Can you work these out from the model? Positions are in its coordinate system, mm. Face numbers are marked on the shaded views. A direction names the side the tool comes from. Give positions to 0.01 mm unless a question says otherwise; leave off trailing zeros. Write each loop counter-clockwise with the first axis right and the second up, starting at its lowest first coordinate (ties: lowest second). Pieces come first, ordered by that corner, then holes. Notation, with made-up numbers: (79, -13.75) -> (127, -13.75) arc R11 ccw to (127, 5.25) -> close; hole circle Ø2 at (-16.5, 34.5). An arc over 180 degrees is marked (long way). Answer as CSV lines item,"result". Start each with the question number.
1. If we mould it in two halves opening along Z, with no side actions, what happens to the marked faces 6, 7, 8 and 9? For each: pulls with the +Z half, pulls with the -Z half, needs draft (parallel to the pull), parting line crosses it, or undercut.
2. If we section it at B-B on y = 3.5: Count the separate pieces of the cut face and the enclosed holes in it, plus the area to 3 significant figures.
3. I'm going to push flat-ended pins straight in: P1, Ø0.8, axis at x = 4, y = 13, coming from the -Z side; P2, Ø2, axis at x = 1, z = 10.5, coming from the +Y side. Where does each tip first touch, or does it pass through?
4. On a 3-axis mill with a long thin cutter (end or side, diameter ignored), from which of +Z, -Z, +X, -X, +Y, -Y can I reach the whole of each face in a straight line? I mean the marked faces 1, 2, 3, 4 and 5. Say none if no direction works.
5. I need wall thicknesses on line 1 (X direction, y = 13.25, z = 11.25) (3 decimals); line 2 (Z direction, x = 18, y = 7); line 3 (Z direction, x = 4, y = 10.5) (1 decimal). Which ranges of each line are inside material? Lowest first, please. Write a range as [from, to].
6. If we section it at A-A on z = 1.75: Write out the boundary of the cut face in (x, y) (3 decimals), plus the area to 3 significant figures.
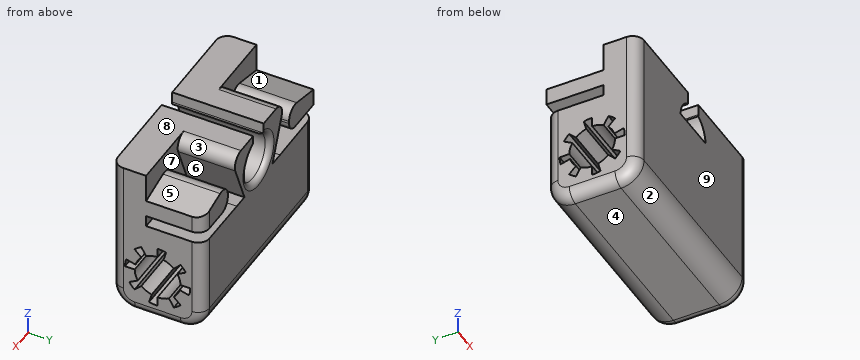
```python
from build123d import *

# Parameters (mm, degrees)
SALIENTE_EXTRUIR1_DEPTH = 16
CROQUIS5_R              = 5.7
CORTAR_EXTRUIR1_DEPTH   = 38
SALIENTE_EXTRUIR2_DEPTH = 0.3
CORTAR_EXTRUIR2_DEPTH   = 10
REDONDEO1_R             = 4
REDONDEO2_R             = 2
REDONDEO3_R             = 1
FILETE1_R               = 2
SALIENTE_EXTRUIR3_START = -36
SALIENTE_EXTRUIR3_DEPTH = 36
PADR_OCIRCULAR1_COUNT   = 8
FILETE2_R               = 2
FILETE3_R               = 2


with BuildPart() as part:
    # Croquis1 → Saliente-Extruir1 (new body)
    with BuildSketch(Plane(origin=(0, 0, 0), x_dir=(1, 0, 0), z_dir=(0, 1, 0))):
        with BuildLine():
            Line((-16.125, 9.1375), (19.875, 9.1375))
            Line((19.875, 9.1375), (19.875, -18.8625))
            Line((19.875, -18.8625), (3.603278106, -18.8625))
            Line((3.603278106, -18.8625), (3.603278106, -16.9125))
            ThreePointArc((3.603278106, -16.9125), (3.593299591, -16.727049938), (3.563479273, -16.543741332))
            ThreePointArc((3.563479273, -16.543741332), (1.875, -8.8125), (0.186520727, -16.543741332))
            ThreePointArc((0.186520727, -16.543741332), (0.156700409, -16.727049938), (0.146721894, -16.9125))
            Line((0.146721894, -16.9125), (0.146721894, -18.8625))
            Line((0.146721894, -18.8625), (-16.125, -18.8625))
            Line((-16.125, -18.8625), (-16.125, 9.1375))
        make_face()
    extrude(amount=SALIENTE_EXTRUIR1_DEPTH)

    # Croquis5 → Cortar-Extruir1 (cut)
    with BuildSketch(Plane(origin=(19.875, 0, 0), x_dir=(0, 0, -1), z_dir=(1, 0, 0))):
        with Locations((0.6375, 8)):
            Circle(CROQUIS5_R)
    extrude(amount=-CORTAR_EXTRUIR1_DEPTH, mode=Mode.SUBTRACT)

    # Croquis8 → Saliente-Extruir2 (add)
    with BuildSketch(Plane.XZ):
        with BuildLine():
            Line((-2.175, 12.8625), (5.925, 12.8625))
            ThreePointArc((5.925, 12.8625), (1.875, 8.8125), (-2.175, 12.8625))
        make_face()
    extrude(amount=-SALIENTE_EXTRUIR2_DEPTH)

    # Croquis9 → Cortar-Extruir2 (cut)
    with BuildSketch(Plane(origin=(0, 16, 0), x_dir=(1, 0, 0), z_dir=(0, 1, 0))):
        Polygon((-8.125, -10.8125), (-8.125, -15.8125), (-16.125, -13.8125), (-16.125, -18.8625), (-6.801553451, -18.8625), (-2.700687259, -8.7125), (-5.179202857, -8.7125), (-16.125, -8.8125), (-16.125, -10.8125), align=None)
    cortar_extruir2 = extrude(amount=-CORTAR_EXTRUIR2_DEPTH, mode=Mode.SUBTRACT)

    # Redondeo1
    redondeo1_edges = [part.edges().sort_by_distance(p)[0] for p in [
        (1.875, 16, -9.1375),
        (1.875, 0, -9.1375),
    ]]
    fillet(redondeo1_edges, radius=REDONDEO1_R)

    # Redondeo2
    redondeo2_edges = [part.edges().sort_by_distance(p)[0] for p in [
        (19.875, 16, 6.8625),
        (-16.125, 16, 1.8375),
        (-16.125, 8, -9.1375),
        (-16.125, 0, 6.8625),
        (-16.125, 1.171572875, -7.965927125),
        (-16.125, 14.828427125, -7.965927125),
        (19.875, 8, -9.1375),
        (19.875, 1.171572875, -7.965927125),
        (19.875, 14.828427125, -7.965927125),
        (19.875, 0, 6.8625),
    ]]
    fillet(redondeo2_edges, radius=REDONDEO2_R)

    # Redondeo3
    redondeo3_edges = [part.edges().sort_by_distance(p)[0] for p in [
        (1.875, 16, 8.8125),
    ]]
    fillet(redondeo3_edges, radius=REDONDEO3_R)

    # Filete1
    filete1_edges = [part.edges().sort_by_distance(p)[0] for p in [
        (-8.125, 11, 10.8125),
        (-8.125, 11, 15.8125),
    ]]
    fillet(filete1_edges, radius=FILETE1_R)

    # Croquis10 → Saliente-Extruir3 (add)
    with BuildSketch(Plane.ZY.offset(16.125).offset(SALIENTE_EXTRUIR3_START)):
        with BuildLine():
            Line((-0.6375, 4), (-0.6375, 2.3))
            ThreePointArc((-0.6375, 2.3), (-2.112768557, 2.49422279), (-3.4875, 3.063655198))
            Line((-3.4875, 3.063655198), (-2.6375, 4.535898385))
            ThreePointArc((-2.6375, 4.535898385), (-1.67277618, 4.136296695), (-0.6375, 4))
        make_face()
    saliente_extruir3 = extrude(amount=SALIENTE_EXTRUIR3_DEPTH)

    # Padr_oCircular1: Saliente-Extruir3 ×8 about axis
    padr_ocircular1_axis = Axis((0, 8, -0.6375), (1, 0, 0))
    for i in range(1, PADR_OCIRCULAR1_COUNT):
        add(saliente_extruir3.rotate(padr_ocircular1_axis, i * 360 / PADR_OCIRCULAR1_COUNT))

    # Filete2
    filete2_edges = [part.edges().sort_by_distance(p)[0] for p in [
        (-6.801553451, 11, 18.8625),
    ]]
    fillet(filete2_edges, radius=FILETE2_R)

    # Espelhar3: Cortar-Extruir2 across plane
    add(cortar_extruir2.mirror(Plane.ZY.offset(-1.875)), mode=Mode.SUBTRACT)

    # Filete3
    filete3_edges = [part.edges().sort_by_distance(p)[0] for p in [
        (11.875, 11, 10.8125),
        (11.875, 11, 15.8125),
        (10.551553451, 11, 18.8625),
    ]]
    fillet(filete3_edges, radius=FILETE3_R)


solid = part.part
```
Computed values:
1,face 6,"undercut"
1,face 7,"undercut"
1,face 8,"pulls with the +Z half"
1,face 9,"needs draft"
2,separate pieces,"3"
2,enclosed holes,"0"
2,area,"871 mm2"
3,P1,"stops at z = -9.09"
3,P2,"stops at y = 0.3"
4,face 1,"+Z, -X, +Y"
4,face 2,"-Z, +X, -X, -Y"
4,face 3,"+X, +Y"
4,face 4,"-Z, +X, -X, +Y, -Y"
4,face 5,"+Z, +X, +Y"
5,line 1,"x = [-16.125, -8.877], [-3.726, -1.84], [5.59, 7.476], [12.627, 19.875]"
5,line 2,"z = [-9.13, -6.25], [3.24, 8.8], [10.81, 14.28]"
5,line 3,"z = [-9.1, -5], [2.5, 9.4], [16.3, 18.9]"
6,outline,"(-16.125, 2) arc R2 ccw to (-14.125, 0) -> (17.875, 0) arc R2 ccw to (19.875, 2) -> (19.875, 4.791) -> (-16.125, 4.791) -> close; (-16.125, 12.135) -> (19.875, 12.135) -> (19.875, 14) arc R2 ccw to (17.875, 16) -> (-14.125, 16) arc R2 ccw to (-16.125, 14) -> close"
6,area,"308 mm2"
